```python
from build123d import *

# Parameters (mm, degrees)
CROQUIS1_R                   = 2.5
SALIENTE_EXTRUIR1_DEPTH      = 5
SALIENTE_EXTRUIR2_DEPTH      = 6
SALIENTE_EXTRUIR5_DEPTH      = 2
SALIENTE_EXTRUIR5_DEPTH_BACK = 0.1
CROQUIS2_W                   = 41.5
CROQUIS2_H                   = 5.75
CROQUIS2_H_2                 = 4
CROQUIS2_H_3                 = 1.75
CROQUIS2_W_2                 = 1.75
CROQUIS3_R                   = 2
SALIENTE_EXTRUIR6_DEPTH      = 8
CORTAR_EXTRUIR1_REACH        = 36.373
CORTAR_EXTRUIR2_START        = -2
CROQUIS4_R                   = 3.000239327
CROQUIS4_R_2                 = 2
CROQUIS4_R_3                 = 3
CORTAR_EXTRUIR2_DEPTH        = 2
REDONDEO1_R                  = 2
REDONDEO2_R                  = 2


with BuildPart() as part:
    # Croquis1 → Saliente-Extruir1 (new body)
    with BuildSketch(Plane(origin=(0, 0, 0), x_dir=(1, 0, 0), z_dir=(0, 1, 0))):
        with BuildLine():
            Line((-22.5, -22.5), (22.5, -22.5))
            Line((22.5, -22.5), (22.5, -20.75))
            Line((22.5, -20.75), (-3.5, -20.75))
            ThreePointArc((-3.5, -20.75), (-7.5, -16.75), (-3.5, -12.75))
            Line((-3.5, -12.75), (22.5, -12.75))
            Line((22.5, -12.75), (22.5, 22.5))
            Line((22.5, 22.5), (-22.5, 22.5))
            Line((-22.5, 22.5), (-22.5, 20.75))
            Line((-22.5, 20.75), (3.5, 20.75))
            ThreePointArc((3.5, 20.75), (7.5, 16.75), (3.5, 12.75))
            Line((3.5, 12.75), (-22.5, 12.75))
            Line((-22.5, 12.75), (-22.5, -22.5))
        make_face()
        with Locations(Location((0, 0, 0), (0, 0, 270))):
            Circle(CROQUIS1_R, mode=Mode.SUBTRACT)
    extrude(amount=-SALIENTE_EXTRUIR1_DEPTH)

    # Croquis1<3> → Saliente-Extruir2 (add)
    with BuildSketch(Plane(origin=(0, 0, 0), x_dir=(1, 0, 0), z_dir=(0, 1, 0))):
        Polygon((-22.5, 7.75), (-22.5, -22.5), (22.5, -22.5), (22.5, -20.75), (-3.5, -20.75), (-20.75, -20.75), (-20.75, 7.75), align=None)
        Polygon((-22.5, 22.5), (-22.5, 20.75), (3.5, 20.75), (20.75, 20.75), (20.75, -7.75), (22.5, -7.75), (22.5, 22.5), align=None)
    extrude(amount=SALIENTE_EXTRUIR2_DEPTH)

    # Croquis2 → Saliente-Extruir5 (add, two sides: drawn at the far end of the back side and taken through both)
    with BuildSketch(Plane(origin=(0, 6, 0), x_dir=(1, 0, 0), z_dir=(0, 1, 0)).offset(-SALIENTE_EXTRUIR5_DEPTH_BACK)):
        with Locations((0, 19.625)):
            Rectangle(CROQUIS2_W, CROQUIS2_H)
        Polygon((-20.75, 22.5), (-22.5, 22.5), (-22.5, 7.75), (-20.75, 7.75), (-20.75, 16.75), align=None)
        with Locations((0, -18.75)):
            Rectangle(CROQUIS2_W, CROQUIS2_H_2)
        with Locations((0, -21.625)):
            Rectangle(CROQUIS2_W, CROQUIS2_H_3)
        Polygon((-20.75, 7.75), (-22.5, 7.75), (-22.5, -22.5), (-20.75, -22.5), (-20.75, -20.75), (-20.75, -16.75), align=None)
        Polygon((22.5, 22.5), (20.75, 22.5), (20.75, 16.75), (20.75, -16.75), (20.75, -20.75), (22.5, -20.75), align=None)
        with Locations((21.625, -21.625)):
            Rectangle(CROQUIS2_W_2, CROQUIS2_H_3)
    extrude(amount=SALIENTE_EXTRUIR5_DEPTH + SALIENTE_EXTRUIR5_DEPTH_BACK)

    # Croquis3 → Saliente-Extruir6 (add)
    with BuildSketch(Plane(origin=(0, 8, 0), x_dir=(1, 0, 0), z_dir=(0, 1, 0))):
        with BuildLine():
            Line((-20.75, 5), (-20.75, -5))
            Line((-20.75, -5), (-17.5, -5))
            Line((-17.5, -5), (-17.5, -2))
            ThreePointArc((-17.5, -2), (-19.5, 0), (-17.5, 2))
            Line((-17.5, 2), (-17.5, 5))
            Line((-17.5, 5), (-20.75, 5))
        make_face()
        with Locations((-17.5, 0)):
            Circle(CROQUIS3_R)
        with BuildLine():
            Line((-17.5, -5), (-17.5, 5))
            ThreePointArc((-17.5, 5), (-12.5, 0), (-17.5, -5))
        make_face()
        with BuildLine():
            ThreePointArc((-17.5, 2), (-19.5, 0), (-17.5, -2))
            Line((-17.5, -2), (-17.5, 2))
        make_face()
        with BuildLine():
            Line((-17.5, 2), (-17.5, -2))
            ThreePointArc((-17.5, -2), (-16.085786438, -1.414213562), (-15.5, 0))
            ThreePointArc((-15.5, 0), (-16.085786438, 1.414213562), (-17.5, 2))
        make_face()
    saliente_extruir6 = extrude(amount=-SALIENTE_EXTRUIR6_DEPTH)

    # Croquis3<3> → Cortar-Extruir1 (cut, up to next)
    with BuildSketch(Plane(origin=(0, 8, 0), x_dir=(1, 0, 0), z_dir=(0, 1, 0)), mode=Mode.PRIVATE) as cortar_extruir1_sk1:
        with BuildLine():
            ThreePointArc((-17.5, 2), (-19.5, 0), (-17.5, -2))
            Line((-17.5, -2), (-17.5, 2))
        make_face()
    cortar_extruir1_tool1 = extrude(cortar_extruir1_sk1.sketch, amount=-CORTAR_EXTRUIR1_REACH, mode=Mode.PRIVATE) & part.part
    # Croquis3<3> → Cortar-Extruir1 (cut, up to next)
    with BuildSketch(Plane(origin=(0, 8, 0), x_dir=(1, 0, 0), z_dir=(0, 1, 0)), mode=Mode.PRIVATE) as cortar_extruir1_sk2:
        with BuildLine():
            Line((-17.5, 2), (-17.5, -2))
            ThreePointArc((-17.5, -2), (-16.085786438, -1.414213562), (-15.5, 0))
            ThreePointArc((-15.5, 0), (-16.085786438, 1.414213562), (-17.5, 2))
        make_face()
    cortar_extruir1_tool2 = extrude(cortar_extruir1_sk2.sketch, amount=-CORTAR_EXTRUIR1_REACH, mode=Mode.PRIVATE) & part.part
    # Croquis3<3> → Cortar-Extruir1 (cut, up to next)
    with BuildSketch(Plane(origin=(0, 8, 0), x_dir=(1, 0, 0), z_dir=(0, 1, 0)), mode=Mode.PRIVATE) as cortar_extruir1_sk3:
        with BuildLine():
            ThreePointArc((-17.5, 2), (-19.5, 0), (-17.5, -2))
            Line((-17.5, -2), (-17.5, 2))
        make_face()
    cortar_extruir1_tool3 = extrude(cortar_extruir1_sk3.sketch, amount=-CORTAR_EXTRUIR1_REACH, mode=Mode.PRIVATE) & part.part
    # Croquis3<3> → Cortar-Extruir1 (cut, up to next)
    with BuildSketch(Plane(origin=(0, 8, 0), x_dir=(1, 0, 0), z_dir=(0, 1, 0)), mode=Mode.PRIVATE) as cortar_extruir1_sk4:
        with BuildLine():
            Line((-17.5, 2), (-17.5, -2))
            ThreePointArc((-17.5, -2), (-16.085786438, -1.414213562), (-15.5, 0))
            ThreePointArc((-15.5, 0), (-16.085786438, 1.414213562), (-17.5, 2))
        make_face()
    cortar_extruir1_tool4 = extrude(cortar_extruir1_sk4.sketch, amount=-CORTAR_EXTRUIR1_REACH, mode=Mode.PRIVATE) & part.part
    cortar_extruir1_1 = cortar_extruir1_tool1.solids().sort_by_distance((-18.348826, 8, 0))[0]
    add(cortar_extruir1_1, mode=Mode.SUBTRACT)
    cortar_extruir1_2 = cortar_extruir1_tool2.solids().sort_by_distance((-16.651174, 8, 0))[0]
    add(cortar_extruir1_2, mode=Mode.SUBTRACT)
    cortar_extruir1_3 = cortar_extruir1_tool3.solids().sort_by_distance((-18.348826, 8, 0))[0]
    add(cortar_extruir1_3, mode=Mode.SUBTRACT)
    cortar_extruir1_4 = cortar_extruir1_tool4.solids().sort_by_distance((-16.651174, 8, 0))[0]
    add(cortar_extruir1_4, mode=Mode.SUBTRACT)
    cortar_extruir1 = cortar_extruir1_1 + cortar_extruir1_2 + cortar_extruir1_3 + cortar_extruir1_4  # Cortar-Extruir1 as one shape, for the pattern or mirror that repeats it

    # Simetría1: Saliente-Extruir6, Cortar-Extruir1 across plane
    add(saliente_extruir6.mirror(Plane(origin=(0, 0, 0), x_dir=(0, 0, 1), z_dir=(1, 0, 0))))
    add(cortar_extruir1.mirror(Plane(origin=(0, 0, 0), x_dir=(0, 0, 1), z_dir=(1, 0, 0))), mode=Mode.SUBTRACT)

    # Croquis4 → Cortar-Extruir2 (cut)
    # profile 1 of 2: a face of its own
    with BuildSketch(Plane.XZ.offset(5).offset(CORTAR_EXTRUIR2_START)):
        with Locations(Location((-17.5, 0, 0), (0, 0, 270))):
            Circle(CROQUIS4_R)
        with Locations(Location((-17.5, 0, 0), (0, 0, 90))):
            Circle(CROQUIS4_R_2, mode=Mode.SUBTRACT)
    # profile 2 of 2: a face of its own
    with BuildSketch(Plane.XZ.offset(5).offset(CORTAR_EXTRUIR2_START)):
        with Locations(Location((17.5, 0, 0), (0, 0, 270))):
            Circle(CROQUIS4_R_3)
        with Locations(Location((17.5, 0, 0), (0, 0, 90))):
            Circle(CROQUIS4_R_2, mode=Mode.SUBTRACT)
    extrude(amount=CORTAR_EXTRUIR2_DEPTH, mode=Mode.SUBTRACT)

    # Redondeo1
    redondeo1_edges = [part.edges().sort_by_distance(p)[0] for p in [
        (20.75, 6.95, 16.75),
        (-20.75, 6.95, 16.75),
        (20.75, 6.95, -16.75),
        (-20.75, 4, -5),
        (-20.75, 4, 5),
        (20.75, 4, 5),
        (20.75, 4, -5),
        (-20.75, 6.95, -16.75),
    ]]
    fillet(redondeo1_edges, radius=REDONDEO1_R)

    # Redondeo2
    redondeo2_edges = [part.edges().sort_by_distance(p)[0] for p in [
        (-22.5, 1.5, -22.5),
        (22.5, 1.5, -22.5),
        (-22.5, 1.5, 22.5),
        (22.5, 1.5, 22.5),
        (20.75, 2.95, -20.75),
        (-20.75, 2.95, 20.75),
    ]]
    fillet(redondeo2_edges, radius=REDONDEO2_R)


solid = part.part
```
Input: part model. Units: mm. Frame: model coordinates. A direction names the side the tool comes from. Round coordinates to 2 decimals unless told otherwise and drop trailing zeros. Loops run counter-clockwise (first coordinate to the right, second up) from the corner with the lowest first, then second, coordinate; pieces in that order, holes last. Notation, with made-up numbers: (-12, 22.5) -> (14, 22.5) arc R25 ccw to (14, 40.5) -> close; hole circle Ø9 at (3, 13). An arc over 180 degrees is marked (long way). One line per item, written item: value.
(1) Section B-B (x = -10). Return the cut outline in (y, z).
Geometry check:
outline: (-5, -22.5) -> (8, -22.5) -> (8, -16.75) -> (5.9, -16.75) -> (5.9, -20.75) -> (-5, -20.75) -> close; (-5, -12.75) -> (0, -12.75) -> (0, 20.75) -> (5.9, 20.75) -> (5.9, 16.75) -> (8, 16.75) -> (8, 22.5) -> (-5, 22.5) -> close
(2) Section A-A (y = 3). Give the number of separate pieces and of enclosed holes in the cut face, plus the area to 3 significant figures.
Geometry check:
separate pieces: 2
enclosed holes: 2
area: 377 mm2
(3) Material intervals for line 1 (X direction, y = -4.2, z = 0); line 2 (Z direction, x = -2.5, y = 3.75); line 3 (Z direction, x = -7, y = 7), sorted ascending. Write a range as [from, to].
Geometry check:
line 1: [-22.5, -20.5], [-14.5, -2.5], [2.5, 14.5], [20.5, 22.5]
line 2: [-22.5, -20.75], [20.75, 22.5]
line 3: [-22.5, -16.75], [16.75, 22.5]
(4) Pin query (flat end, axial travel): pin 1 (4 mm diameter, centred on x = -12.5, z = 14, fed in from +Y); pin 2 (0.9 mm diameter, centred on x = -22, y = 4, fed in from -Z). Return the tip coordinate at first contact, or that it passes through.
Geometry check:
pin 1: y = 0
pin 2: z = -22.2
(5) Section C-C (z = 10). Return the cut outline in (x, y).
Geometry check:
outline: (-22.5, -5) -> (22.5, -5) -> (22.5, 0) -> (-20.75, 0) -> (-20.75, 8) -> (-22.5, 8) -> close; (20.75, 5.9) -> (22.5, 5.9) -> (22.5, 8) -> (20.75, 8) -> close
(6) Mould query, pull axis X, two halves, no side actions, for faces 5 (the face through (-7.5, -2.5, 16.8)), 6 (the face through (20.75, 4, -13)), 7 (the face through (-22, 3, -7.75)). Classes: pulls with the +X half, pulls with the -X half, needs draft (parallel to the pull), parting line crosses it, or undercut.
Geometry check:
face 5: pulls with the +X half
face 6: undercut
face 7: needs draft
(7) Section D-D (x = 0). Return the cut outline in (y, z).
Geometry check:
outline: (-5, -22.5) -> (8, -22.5) -> (8, -16.75) -> (5.9, -16.75) -> (5.9, -20.75) -> (-5, -20.75) -> close; (-5, -12.75) -> (0, -12.75) -> (0, -2.5) -> (-5, -2.5) -> close; (-5, 2.5) -> (0, 2.5) -> (0, 12.75) -> (-5, 12.75) -> close; (-5, 20.75) -> (5.9, 20.75) -> (5.9, 16.75) -> (8, 16.75) -> (8, 22.5) -> (-5, 22.5) -> close
(8) Set-up query: faces 1 (the face through (-15.47, -3.99, 2.21)), 2 (the face through (-3, 5.9, -18)), 3 (the face through (22, 3, 7.75)), 4 (the face through (0, 7, -16.75)). Return all of +Z, -Z, +X, -X, +Y, -Y with unobstructed straight access to the full face (end or side cutting, diameter ignored); none if empty.
Geometry check:
face 1: -Y
face 2: -X
face 3: +X
face 4: +Y
